from build123d import *

# Parameters (mm, degrees)
EXTRUDE_1_DEPTH     = 4
SKETCH_2_W          = 2.925
SKETCH_2_H          = 50
EXTRUDE_2_DEPTH     = 7
SKETCH_3_R          = 1.6
CUT_EXTRUDE_1_DEPTH = 42.596273872
CHAMFER_1_SIZE      = 0.5
FILLET_1_R          = 6


with BuildPart() as part:
    # 草图1 → 凸台-拉伸1 (new body)
    with BuildSketch(Plane(origin=(0, 0, 0), x_dir=(1, 0, 0), z_dir=(0, 1, 0))):
        Polygon((-10.5, 25), (12.5, 25), (12.5, 12.5), (32.5, 12.5), (32.5, -12.5), (12.5, -12.5), (12.5, -25), (-10.5, -25), align=None)
    extrude(amount=EXTRUDE_1_DEPTH)

    # 草图2 → 凸台-拉伸2 (add)
    with BuildSketch(Plane(origin=(0, 4, 0), x_dir=(1, 0, 0), z_dir=(0, 1, 0))):
        Polygon((7.575, -25), (7.575, -7.575), (32.5, -7.575), (32.5, -12.5), (12.5, -12.5), (12.5, -25), align=None)
        Polygon((32.5, 7.575), (7.575, 7.575), (7.575, 25), (12.5, 25), (12.5, 12.5), (32.5, 12.5), align=None)
        with Locations((-9.0375, 0)):
            Rectangle(SKETCH_2_W, SKETCH_2_H)
    extrude(amount=EXTRUDE_2_DEPTH)

    # 草图3 → 切除-拉伸1 (cut, through all)
    with BuildSketch(Plane(origin=(0, 4, 0), x_dir=(1, 0, 0), z_dir=(0, 1, 0))):
        with Locations(Location((0, 0, 0), (0, 0, 270))):
            Circle(SKETCH_3_R)
        with Locations(Location((0, 20, 0), (0, 0, 270))):
            Circle(SKETCH_3_R)
        with Locations(Location((0, -20, 0), (0, 0, 270))):
            Circle(SKETCH_3_R)
        with Locations(Location((27.5, 0, 0), (0, 0, 270))):
            Circle(SKETCH_3_R)
    extrude(amount=-CUT_EXTRUDE_1_DEPTH, mode=Mode.SUBTRACT)

    # 倒角1
    chamfer_1_edges = [part.edges().sort_by_distance(p)[0] for p in [
        (7.575, 7.5, 7.575),
        (20.0375, 11, 7.575),
        (7.575, 11, 16.2875),
        (7.575, 7.5, -7.575),
        (7.575, 11, -16.2875),
        (20.0375, 11, -7.575),
        (-7.575, 11, 0),
    ]]
    chamfer(chamfer_1_edges, length=CHAMFER_1_SIZE)

    # 圆角1
    fillet_1_edges = [part.edges().sort_by_distance(p)[0] for p in [
        (12.5, 5.5, 12.5),
        (12.5, 5.5, -12.5),
    ]]
    fillet(fillet_1_edges, radius=FILLET_1_R)


solid = part.part
The listing builds one solid part. Answer for the finished solid, in the listing's coordinates (mm). A direction names the side the tool comes from. Coordinates: 2 decimals unless noted, no trailing zeros. Order: outer loops, then holes, each group sorted by start corner. A loop starts at its lowest first (then second) coordinate and runs counter-clockwise, first axis right, second up. Notation, with made-up numbers: M 54.25,-8.75 L 64.25,-8.75 A21 ccw 64.25,20.25 Z; hole C -26.75,-34 d8. An arc over 180 degrees is marked long. Use CSV: the item, a comma, the result in double quotes.
Q1. Given pin 1 Ø1.5 at (x, z) = (25, -7) entering from +Y (3 decimals); pin 2 Ø4 at (x, z) = (6.5, 7.5) entering from -Y; pin 3 Ø4 at (x, z) = (-2, -2.5) entering from +Y; pin 4 Ø5.5 at (x, y) = (26.5, 3) entering from -Z, each flat-ended and moving along its own axis, determine where each tip first touches the part or whether it passes through.
Here are the results:
pin 1,"y = 10.675"
pin 2,"y = 0"
pin 3,"y = 4"
pin 4,"z = -12.5"
Q2. Section A-A (y = 8) is taken. Determine the outline of the cut face in (x, z) (3 decimals), then the cut area to 3 significant figures.
Here are the results:
outline,"M -10.5,-25 L -7.575,-25 L -7.575,25 L -10.5,25 Z; M 7.575,-25 L 12.5,-25 L 12.5,-18.5 A6 cw 18.5,-12.5 L 32.5,-12.5 L 32.5,-7.575 L 8.075,-7.575 L 7.575,-8.075 Z; M 7.575,8.075 L 8.075,7.575 L 32.5,7.575 L 32.5,12.5 L 18.5,12.5 A6 cw 12.5,18.5 L 12.5,25 L 7.575,25 Z"
area,"530 mm2"
Q3. Determine the mould class of faces 1 (the flat face through (12.5, 5, -22)), 2 (the flat face through (1, 3, 25)), 3 (the flat face through (8, 4, 0)) for opening direction X: pulls with the +X half, pulls with the -X half, needs draft (parallel to the pull), parting line crosses it, or undercut.
Here are the results:
face 1,"pulls with the +X half"
face 2,"needs draft"
face 3,"undercut"
Q4. Section D-D (y = 1) is taken. Determine the outline of the cut face in (x, z).
Here are the results:
outline,"M -10.5,-25 L 12.5,-25 L 12.5,-18.5 A6 cw 18.5,-12.5 L 32.5,-12.5 L 32.5,12.5 L 18.5,12.5 A6 cw 12.5,18.5 L 12.5,25 L -10.5,25 Z; hole C 0,-20 d3.2; hole C 0,0 d3.2; hole C 0,20 d3.2; hole C 27.5,0 d3.2"
Q5. Section B-B (z = 20) is taken. Determine the outline of the cut face in (x, y) (3 decimals), then the cut area to 3 significant figures.
Here are the results:
outline,"M -10.5,0 L -1.6,0 L -1.6,4 L -7.575,4 L -7.575,10.5 L -8.075,11 L -10.5,11 Z; M 1.6,0 L 12.5,0 L 12.5,11 L 8.075,11 L 7.575,10.5 L 7.575,4 L 1.6,4 Z"
area,"134 mm2"
Q6. A tool of negligible diameter and unlimited length cuts with its end or side. For faces 4 (the cylindrical face through (1.08, 2.03, 18.82)), 5 (the flat face through (20, 7, -7.575)), 6 (the flat face through (7.575, 7, -16)), 7 (the flat face through (25, 5, -12.5)), 8 (the flat face through (26, 5, 12.5)), from which of +Z, -Z, +X, -X, +Y, -Y can it reach the whole face along a straight path? Write none if from no direction.
Here are the results:
face 4,"+Y, -Y"
face 5,"+X, +Y"
face 6,"+Z, -Z, +Y"
face 7,"-Z, +X, +Y, -Y"
face 8,"+Z, +X, +Y, -Y"
Q7. Section C-C (x = 0) is taken. Determine the outline of the cut face in (y, z), then the cut area to 3 significant figures.
Here are the results:
outline,"M 0,-25 L 4,-25 L 4,-21.6 L 0,-21.6 Z; M 0,-18.4 L 4,-18.4 L 4,-1.6 L 0,-1.6 Z; M 0,1.6 L 4,1.6 L 4,18.4 L 0,18.4 Z; M 0,21.6 L 4,21.6 L 4,25 L 0,25 Z"
area,"162 mm2"
Q8. Straight lines are drawn through the part: L1, parallel to X at y = 2.2, z = 0; L2, parallel to Z at x = 25.5, y = 6 (3 decimals); L3, parallel to X at y = 4.75, z = -11.5 (3 decimals). For each, find the intervals that lie inside material, in ascending order.
Here are the results:
L1,"-10.5 to -1.6, 1.6 to 25.9, 29.1 to 32.5"
L2,"-12.5 to -7.575, 7.575 to 12.5"
L3,"-10.5 to -7.575, 7.575 to 32.5"
